Geometry: final body of the model. Coordinates: model frame, mm. Coordinates: 2 decimals unless noted, no trailing zeros. Write each loop counter-clockwise with the first axis right and the second up, starting at its lowest first coordinate (ties: lowest second). Pieces come first, ordered by that corner, then holes.
Autodesk Inventor part; units mm, degrees
ref_plane "YZ Plane" through (0, 0, 0) normal (1, 0, 0) x (0, 1, 0)
ref_plane "XZ Plane" through (0, 0, 0) normal (0, 1, 0) x (-1, 0, 0)
ref_plane "XY Plane" through (0, 0, 0) normal (0, 0, 1) x (1, 0, 0)
sketch "Sketch1" plane through (0, 0, 0) normal (0, 0, 1) x (1, 0, 0)
  line L0 (270.51, 284.48) -> (-270.51, -284.48) construction
  line L1 (-270.51, 284.48) -> (270.51, -284.48) construction
  line L2 (-270.51, -284.48) -> (-257.81, -284.48)
  line L3 (-207.01, -284.48) -> (207.01, -284.48)
  line L4 (257.81, -284.48) -> (270.51, -284.48)
  line L5 (270.51, -284.48) -> (270.51, 203.2)
  line L6 (207.005, 284.48) -> (-207.015, 284.48)
  line L7 (-207.015, 206.375) -> (-207.015, 284.48)
  line L8 (-210.185, 203.2) -> (-270.51, 203.2)
  line L9 (-270.51, 203.2) -> (-270.51, -284.48)
  arc A0 (-210.185, 203.2) -> (-207.015, 206.375) centre (-210.19, 206.375) ccw
  line L10 (207.005, 284.48) -> (207.005, 206.375)
  line L11 (270.51, 203.2) -> (210.185, 203.2)
  arc A1 (207.005, 206.375) -> (210.185, 203.2) centre (210.18, 206.375) ccw
  line L12 (-257.81, -284.48) -> (-257.81, -206.375)
  line L13 (-207.01, -284.48) -> (-207.01, -206.375)
  arc A2 (-254.635, -203.2) -> (-257.81, -206.375) centre (-254.635, -206.375) ccw
  arc A3 (-207.01, -206.375) -> (-210.185, -203.2) centre (-210.185, -206.375) ccw
  line L14 (-254.635, -203.2) -> (-210.185, -203.2)
  line L15 (207.01, -284.48) -> (207.01, -206.375)
  line L16 (257.81, -284.48) -> (257.81, -206.375)
  arc A4 (210.185, -203.2) -> (207.01, -206.375) centre (210.185, -206.375) ccw
  arc A5 (257.81, -206.375) -> (254.635, -203.2) centre (254.635, -206.375) ccw
  line L17 (210.185, -203.2) -> (254.635, -203.2)
  point P0 (0, 0)
  point P1 (0, 0)
  dimension "d0" = 541.02
  dimension "d1" = 568.96
  dimension "d2" = 12.7
  dimension "d6" = 414.02
  dimension "d10" = 12.7
  dimension "d11" = 487.68
  dimension "d14" = 414.02
  dimension "d19" = 78.105
  dimension "d20" = 60.325
  dimension "d22" = 78.105
  dimension "d23" = 60.325
  dimension "d26" = 78.105
  dimension "d27" = 78.105
  dimension "d28" = 44.45
  dimension "d29" = 50.8
  dimension "d30" = 78.105
  dimension "d31" = 78.105
extrude "Extrusion1" add sketch "Sketch1" along normal blind 3.175
properties part number "BK-BKT120-BasePlateextruded" material "Aluminum 6061"
Item 1: Section A-A, the plane z = 0.65. Output: boundary loops of the cut face in (x, y) (3 decimals), plus the area to 3 significant figures.
Derived:
outline: (-270.51, -284.48) - (-257.81, -284.48) - (-257.81, -206.375) arc R3.175 cw to (-254.635, -203.2) - (-210.185, -203.2) arc R3.175 cw to (-207.01, -206.375) - (-207.01, -284.48) - (207.01, -284.48) - (207.01, -206.375) arc R3.175 cw to (210.185, -203.2) - (254.635, -203.2) arc R3.175 cw to (257.81, -206.375) - (257.81, -284.48) - (270.51, -284.48) - (270.51, 203.2) - (210.185, 203.2) arc R3.175 cw to (207.005, 206.375) - (207.005, 284.48) - (-207.015, 284.48) - (-207.015, 206.375) arc R3.175 cw to (-210.185, 203.2) - (-270.51, 203.2) - close
area: 289,000 mm2
Item 2: Section B-B, the plane y = 232.5. Output: boundary loops of the cut face in (x, z) (3 decimals), plus the area to 3 significant figures.
Derived:
outline: (-207.015, 0) - (207.005, 0) - (207.005, 3.175) - (-207.015, 3.175) - close
area: 1,310 mm2
Item 3: Material intervals for probe 1 along X at (y, z) = (220, 2.3) (3 decimals); probe 2 along Y at (x, z) = (242, 2.9), sorted ascending.
Derived:
probe 1: x = -207.015 to 207.005
probe 2: y = -203.2 to 203.2
Item 4: Pin query (flat end, axial travel): pin 1 (6 mm diameter, centred on x = -80, y = -101, fed in from -Z); pin 2 (1 mm diameter, centred on x = -227.5, z = 1.5, fed in from -Y); pin 3 (1.6 mm diameter, centred on x = 227, z = 1, fed in from +Y); pin 4 (1.6 mm diameter, centred on y = 261, z = 2.5, fed in from +X) (3 decimals). Return the tip coordinate at first contact, or that it passes through.
Derived:
pin 1: stops at z = 0
pin 2: stops at y = -203.2
pin 3: stops at y = 203.2
pin 4: stops at x = 207.005
